Check sheet for the modelled part. Datum: model origin and axes. Units: mm. Face numbers are marked on the shaded views. A direction names the side the tool comes from. Give positions to 0.01 mm unless a question says otherwise; leave off trailing zeros. Order: outer loops, then holes, each group sorted by start corner. A loop starts at its lowest first (then second) coordinate and runs counter-clockwise, first axis right, second up. Notation, with made-up numbers: (69.25, 65) -> (93.25, 65) arc R11 ccw to (93.25, 73) -> close; hole circle Ø2 at (43.5, 69). An arc over 180 degrees is marked (long way). Answer in a Markdown table with one row per item. Add a question column.
(1) Cross-section at A-A (x = -1.5). Record the cut outline in (y, z) (3 decimals).
(2) Set-up check for the marked faces 1 and 2: record each of +Z, -Z, +X, -X, +Y, -Y from which the full face is reachable in a straight line by a thin tool's end or side.
(3) Cross-section at B-B (y = 0). Record the cut outline in (x, z), then the cut area to 3 significant figures.
(4) Thickness scan on L1, parallel to X at y = 0.5, z = -4.5; L2, parallel to X at y = -3.5, z = 1.5; L3, parallel to Y at x = 13.5, z = 1.25. Record the ranges inside material, lowest first. Write a range as [from, to].
(5) Go/stop test with flat-tipped pins: pin 1 (1.5 mm diameter, centred on x = 2, y = -2.5, fed in from +Z); pin 2 (5 mm diameter, centred on x = 5.5, z = -3.5, fed in from +Y); pin 3 (6 mm diameter, centred on x = 13, y = -1.5, fed in from +Z). Record where each tip stops, or that it passes through.
(6) Cross-section at C-C (x = 11.5). Record the cut outline in (y, z).
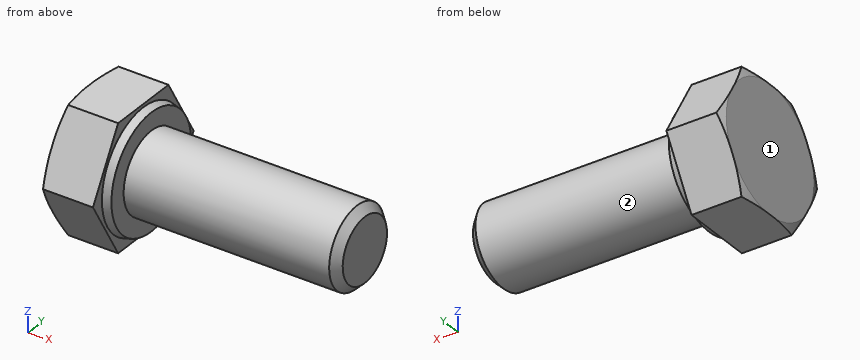
```python
from build123d import *

# Parameters (mm, degrees)
SKETCH_2_OUTSIDE_W  = 18.046
SKETCH_2_OUTSIDE_H  = 18.046
CUT_EXTRUDE_1_DEPTH = 22.994658442
CHAMFER_1_SIZE      = 0.6


with BuildPart() as part:
    # Эскиз1 → Повернуть1 (revolve)
    with BuildSketch(Plane.XY, mode=Mode.PRIVATE) as revolve_1_sk:
        Polygon((-4, 0), (-4, 5.45), (0, 5.45), (0, 4.483974596), (0.6, 4.323205081), (0.6, 3), (16.6, 3), (16.6, 0), align=None)
    revolve(revolve_1_sk.sketch.rotate(Axis((-1000, 0, 0), (1, 0, 0)), 90), axis=Axis((-1000, 0, 0), (1, 0, 0)))

    # Эскиз2 outside → Вырез-Вытянуть1 (cut, through all)
    with BuildSketch(Plane.ZY.offset(4)):
        Rectangle(SKETCH_2_OUTSIDE_W, SKETCH_2_OUTSIDE_H)
        Polygon((0, -5.45), (4.719838451, -2.725), (4.719838451, 2.725), (0, 5.45), (-4.719838451, 2.725), (-4.719838451, -2.725), align=None, mode=Mode.SUBTRACT)
    extrude(amount=-CUT_EXTRUDE_1_DEPTH, mode=Mode.SUBTRACT)

    # Эскиз4 → Вырез-Повернуть1 (revolve, cut)
    with BuildSketch(Plane.XY):
        Polygon((-4, 4.75), (-3.745220836, 5.45), (-4, 5.45), align=None)
    revolve(axis=Axis((-1000, 0, 0), (1, 0, 0)), mode=Mode.SUBTRACT)

    # Фаска1
    chamfer_1_edges = [part.edges().sort_by_distance(p)[0] for p in [
        (16.6, 0, -3),
    ]]
    chamfer(chamfer_1_edges, length=CHAMFER_1_SIZE)


solid = part.part
```
Answer below:
| question | item | result |
|---|---|---|
| 1 | outline | (-5.45, 0) -> (-2.725, -4.72) -> (2.725, -4.72) -> (5.45, 0) -> (2.725, 4.72) -> (-2.725, 4.72) -> close |
| 2 | face 1 | +Z, -Z, -X, +Y, -Y |
| 2 | face 2 | +X |
| 3 | outline | (-4, -4.72) -> (0, -4.72) -> (0, -4.48) -> (0.6, -4.32) -> (0.6, -3) -> (16, -3) -> (16.6, -2.4) -> (16.6, 2.4) -> (16, 3) -> (0.6, 3) -> (0.6, 4.32) -> (0, 4.48) -> (0, 4.72) -> (-4, 4.72) -> close |
| 3 | area | 139 mm² |
| 4 | L1 | x = [-4, 0] |
| 4 | L2 | x = [-4, 0.6] |
| 4 | L3 | y = [-2.73, 2.73] |
| 5 | pin 1 | stops at z = 2.44 |
| 5 | pin 2 | stops at y = 2.83 |
| 5 | pin 3 | stops at z = 3 |
| 6 | outline | circle Ø6 at (0, 0) |
